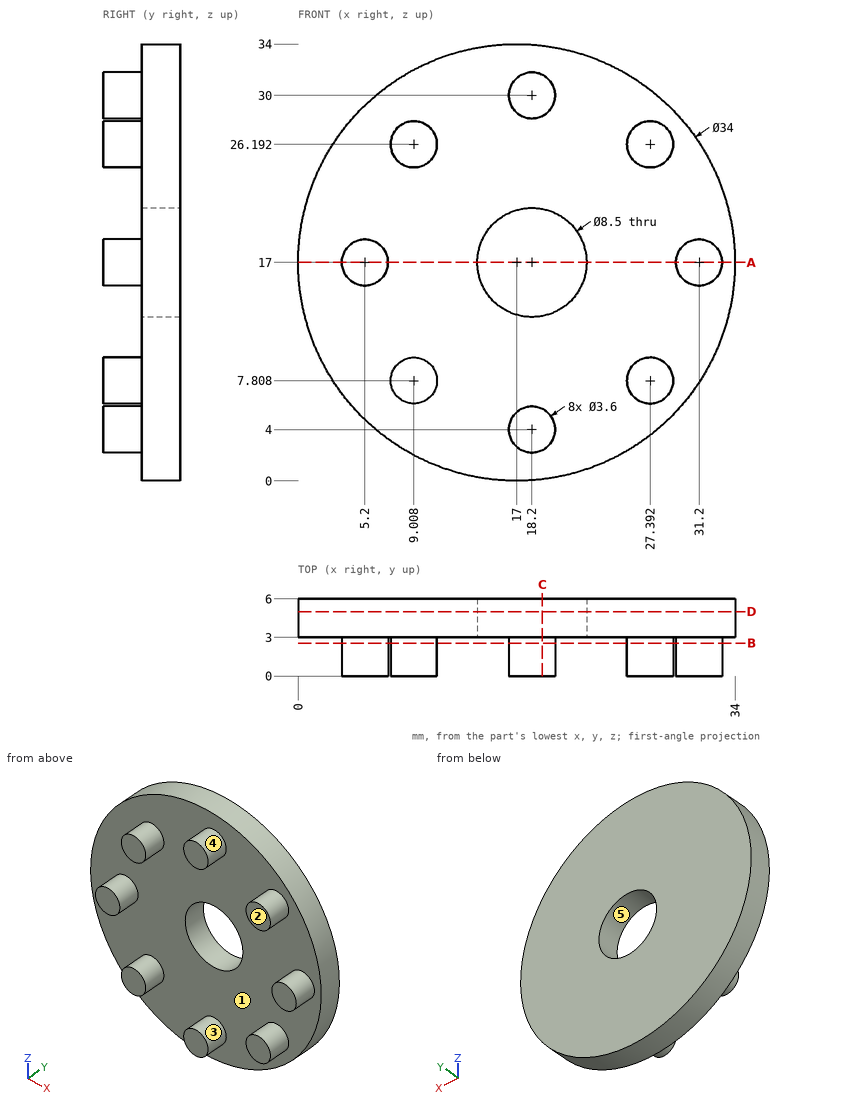
Design review of the part shown in the three views and the two pictorial views. Dimensions are in mm from the part's minimum x, y and z. A direction names the side the tool comes from. Give positions to 0.01 mm unless a question says otherwise; leave off trailing zeros. Order: outer loops, then holes, each group sorted by start corner. A loop starts at its lowest first (then second) coordinate and runs counter-clockwise, first axis right, second up. Notation, with made-up numbers: M 25.5,22.5 L 81.5,22.5 A14 cw 81.5,44.5 Z; hole C 83.5,28 d10. An arc over 180 degrees is marked long. Answer in a Markdown table with one row per item. Add a question column.
(1) Consider section B-B on y = 2.55. State the section outline as (x, z) points.
(2) For pin 1 (1.5 mm diameter, centred on x = 30.5, y = 2.5, fed in from +Z) (1 decimal); pin 2 (5 mm diameter, centred on x = 13.5, z = 27.5, fed in from -Y), all flat-tipped, find the tip position at first contact; note any pin that passes through.
(3) Wall thickness on probe 1 along X at (y, z) = (5.15, 17); probe 2 along Y at (x, z) = (16, 30); probe 3 along X at (y, z) = (2.55, 30): over which ranges is each line inside the solid? List them lowest first. Write a range as [from, to].
(4) Mouldability with a two-part tool opening along X and no side actions: class the marked faces 1, 2 and 3 as +X half, -X half, draft (parallel to the pull), parting line (faces both ways), or undercut.
(5) Consider section C-C on x = 19. State the section outline as (y, z) points.
(6) Consider section A-A on z = 17. State the section outline as (x, y) points.
(7) For the marked faces 4 and 5, list the 3-axis set-ups (+Z, -Z, +X, -X, +Y, -Y) from which the entire face can be reached by the end or side of a thin tool; tool diameter is ignored.
(8) Consider section D-D on y = 5. State the section outline as (x, z) points.
Evaluation:
| question | item | result |
|---|---|---|
| 1 | outline | C 5.2,17 d3.6; C 9.01,7.81 d3.6; C 9.01,26.19 d3.6; C 18.2,4 d3.6; C 18.2,30 d3.6; C 27.39,7.81 d3.6; C 27.39,26.19 d3.6; C 31.2,17 d3.6 |
| 2 | pin 1 | stops at z = 28 |
| 2 | pin 2 | stops at y = 3 |
| 3 | probe 1 | x = [0, 13.95], [22.45, 34] |
| 3 | probe 2 | y = [3, 6] |
| 3 | probe 3 | x = [16.4, 20] |
| 4 | face 1 | undercut |
| 4 | face 2 | draft |
| 4 | face 3 | parting line |
| 5 | outline | M 0,2.39 L 3,2.39 L 3,0.12 L 6,0.12 L 6,12.83 L 3,12.83 L 3,5.61 L 0,5.61 Z; M 0,28.39 L 3,28.39 L 3,21.17 L 6,21.17 L 6,33.88 L 3,33.88 L 3,31.61 L 0,31.61 Z |
| 6 | outline | M 0,3 L 3.4,3 L 3.4,0 L 7,0 L 7,3 L 13.95,3 L 13.95,6 L 0,6 Z; M 22.45,3 L 29.4,3 L 29.4,0 L 33,0 L 33,3 L 34,3 L 34,6 L 22.45,6 Z |
| 7 | face 4 | -Y |
| 7 | face 5 | +Y, -Y |
| 8 | outline | C 17,17 d34; hole C 18.2,17 d8.5 |
